Build history of the part. All positions in model axes, mm. A direction names the side the tool comes from. Give positions to 0.01 mm unless a question says otherwise; leave off trailing zeros. Order: outer loops, then holes, each group sorted by start corner. A loop starts at its lowest first (then second) coordinate and runs counter-clockwise, first axis right, second up. Notation, with made-up numbers: (-27, 63) -> (4, 63) arc R20 ccw to (4, 93) -> close; hole circle Ø5 at (6, -17.75). An arc over 180 degrees is marked (long way). One line per item, written item: value. Start each with the question number.
(1) Probe line 1 (X direction, y = 4.5, z = 11); line 2 (Z direction, x = 13, y = 2.75); line 3 (Y direction, x = 3.75, z = 15.5). List the from-to ranges inside material, lowest first.
(2) Which spindle directions (+Z, -Z, +X, -X, +Y, -Y) get a long thin tool onto all of the face, cutting with end or side? Do faces 5 (the flat face through (12, 0, 11)), 6 (the flat face through (20.5, 5, 11)), 7 (the flat face through (14.6, 4.4, 21.6)). Say none if no direction does.
(3) Pin check, flat tips, straight feed: pin 1 (0.8 mm diameter, centred on x = 4, z = 11, fed in from +Y); pin 2 (2.5 mm diameter, centred on x = 3, y = 5.5, fed in from +Z). Stop position of each tip, or through.
(4) Two-plate mould, pull along X, no slides. Class faces 1 (the flat face through (13, 4, 21.2)), 2 (the flat face through (21, 4, 21.2)), 3 (the flat face through (2, 7.7, 11)), 4 (the flat face through (0, 4, 11)): +X half, -X half, draft (parallel to the pull), parting line (faces both ways), or undercut.
(5) Saw through at C-C on z = 5.75. Give the cut face in (x, y), plus the area to 3 significant figures.
(6) Saw through at B-B on y = 1.75. Give the cut face in (x, z), plus the area to 3 significant figures.
(7) Saw through at D-D on x = 12. Give the cut face in (y, z), plus the area to 3 significant figures.
(8) Saw through at A-A on y = 6.75. Give the cut face in (x, z).
```python
from build123d import *

# Parameters (mm, degrees)
SKETCH_W               = 24
SKETCH_H               = 7.7
PAD_DEPTH              = 22
SKETCH001_W            = 5.2
SKETCH001_H            = 6.5
POCKET_DEPTH           = 0.8
LINEARPATTERN_COUNT    = 3
LINEARPATTERN_PITCH    = 8
SKETCH002_W            = 1
SKETCH002_H            = 5.4
POCKET001_DEPTH        = 22
LINEARPATTERN001_COUNT = 3
LINEARPATTERN001_PITCH = 8


with BuildPart() as part:
    # Sketch → Pad (new body)
    with BuildSketch(Plane.XY):
        with Locations((12, 3.85)):
            Rectangle(SKETCH_W, SKETCH_H)
    extrude(amount=PAD_DEPTH)

    # Sketch001 (on Face6 of Pad) → Pocket (cut)
    with BuildSketch(Plane.XY.offset(22)):
        with Locations((4, 4.45)):
            Rectangle(SKETCH001_W, SKETCH001_H)
    pocket = extrude(amount=-POCKET_DEPTH, mode=Mode.SUBTRACT)

    # LinearPattern: Pocket ×3
    with Locations(*[(i * LINEARPATTERN_PITCH, 0, 0) for i in range(1, LINEARPATTERN_COUNT)]):
        add(pocket, mode=Mode.SUBTRACT)

    # Sketch002 (on Face16 of LinearPattern) → Pocket001 (cut)
    with BuildSketch(Plane.XY.offset(21.2)):
        with Locations((4, 5)):
            Rectangle(SKETCH002_W, SKETCH002_H)
    pocket001 = extrude(amount=-POCKET001_DEPTH, mode=Mode.SUBTRACT)

    # LinearPattern001: Pocket001 ×3
    with Locations(*[(i * LINEARPATTERN001_PITCH, 0, 0) for i in range(1, LINEARPATTERN001_COUNT)]):
        add(pocket001, mode=Mode.SUBTRACT)


solid = part.part
```
Results below:
1. line 1: x = 0 to 3.5, 4.5 to 11.5, 12.5 to 19.5, 20.5 to 24
1. line 2: z = 0 to 21.2
1. line 3: y = 0 to 2.3
2. face 5: +Z, -Z, +X, -X, -Y
2. face 6: +Z, -Z, +Y
2. face 7: +Z, +Y
3. pin 1: stops at y = 2.3
3. pin 2: stops at z = 21.2
4. face 1: undercut
4. face 2: undercut
4. face 3: draft
4. face 4: -X half
5. outline: (0, 0) -> (24, 0) -> (24, 7.7) -> (20.5, 7.7) -> (20.5, 2.3) -> (19.5, 2.3) -> (19.5, 7.7) -> (12.5, 7.7) -> (12.5, 2.3) -> (11.5, 2.3) -> (11.5, 7.7) -> (4.5, 7.7) -> (4.5, 2.3) -> (3.5, 2.3) -> (3.5, 7.7) -> (0, 7.7) -> close
5. area: 169 mm²
6. outline: (0, 0) -> (24, 0) -> (24, 22) -> (22.6, 22) -> (22.6, 21.2) -> (17.4, 21.2) -> (17.4, 22) -> (14.6, 22) -> (14.6, 21.2) -> (9.4, 21.2) -> (9.4, 22) -> (6.6, 22) -> (6.6, 21.2) -> (1.4, 21.2) -> (1.4, 22) -> (0, 22) -> close
6. area: 516 mm²
7. outline: (0, 0) -> (2.3, 0) -> (2.3, 21.2) -> (1.2, 21.2) -> (1.2, 22) -> (0, 22) -> close
7. area: 49.7 mm²
8. outline: (0, 0) -> (3.5, 0) -> (3.5, 21.2) -> (1.4, 21.2) -> (1.4, 22) -> (0, 22) -> close; (4.5, 0) -> (11.5, 0) -> (11.5, 21.2) -> (9.4, 21.2) -> (9.4, 22) -> (6.6, 22) -> (6.6, 21.2) -> (4.5, 21.2) -> close; (12.5, 0) -> (19.5, 0) -> (19.5, 21.2) -> (17.4, 21.2) -> (17.4, 22) -> (14.6, 22) -> (14.6, 21.2) -> (12.5, 21.2) -> close; (20.5, 0) -> (24, 0) -> (24, 22) -> (22.6, 22) -> (22.6, 21.2) -> (20.5, 21.2) -> close
